Source: three-view drawing plus pictorial views. Frame: mm from the lowest corner of the part. Give positions to 0.01 mm unless a question says otherwise; leave off trailing zeros. Write each loop counter-clockwise with the first axis right and the second up, starting at its lowest first coordinate (ties: lowest second). Pieces come first, ordered by that corner, then holes. Notation, with made-up numbers: (77, -11) -> (81, -11) arc R18 cw to (81, 0) -> close; hole circle Ø2 at (50, 70). An arc over 180 degrees is marked (long way). Answer in a Markdown table with one row per item. Add a question column.
Item 1: Section query A-A on z = 100. Output: boundary loops of the cut face in (x, y), plus the area to 3 significant figures.
Item 2: Section query B-B on x = 114. Output: boundary loops of the cut face in (y, z).
Item 3: Section query C-C on y = 3.5. State how many separate pieces and enclosed holes the cut face has, plus the area to 3 significant figures.
Item 4: First-contact query: P1, Ø1.9, axis at y = 9.5, z = 195.5, coming from the -X side; P2, Ø1.5, axis at y = 6, z = 163, coming from the +X side; P3, Ø2, axis at y = 3.5, z = 147, coming from the +X side; P4, Ø6, axis at x = 37.27, z = 12.5, coming from the -Y side. Flat tips, straight axial feed; report the tip coordinate or a pass-through.
Item 5: Section query D-D on x = 76.5. Output: boundary loops of the cut face in (y, z).
Item 6: Material intervals for probe 1 along Z at (x, y) = (28, 5.5); probe 2 along Z at (x, y) = (114, 3.75); probe 3 along X at (y, z) = (9, 100), sorted ascending. Write a range as from..to.
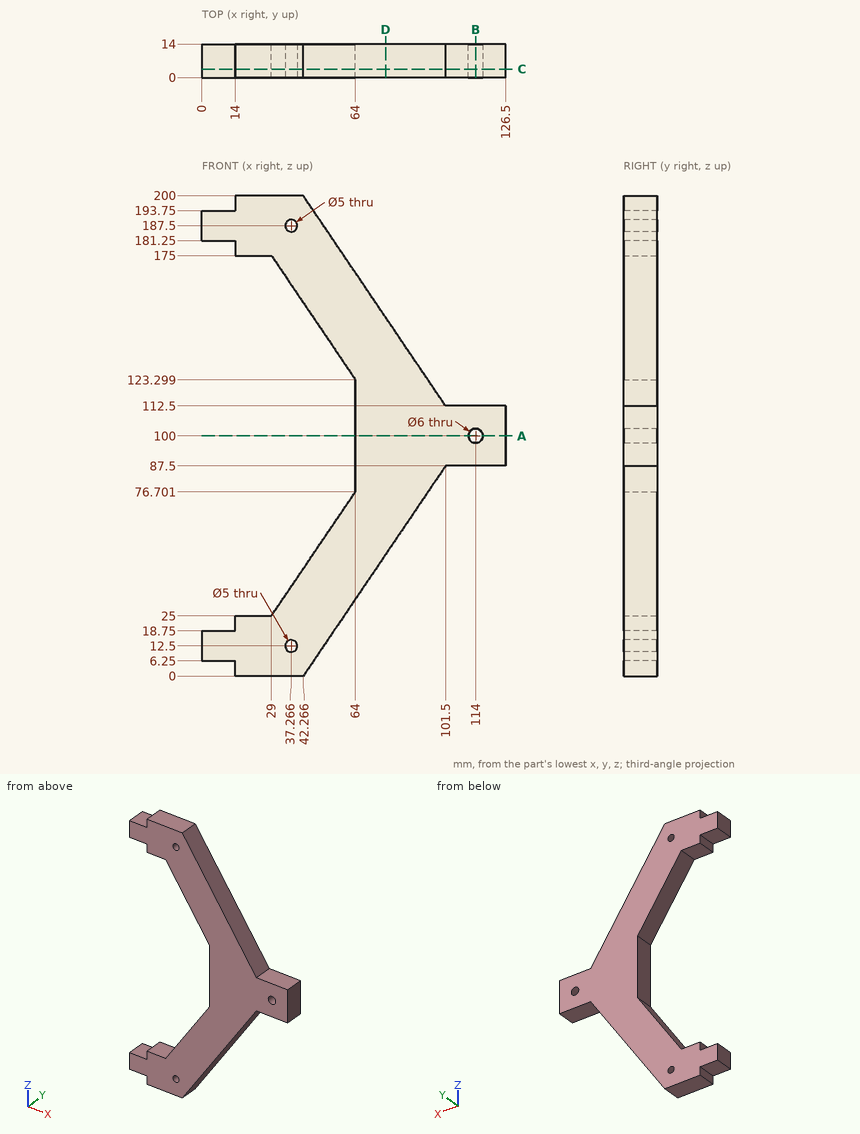
Findings below:
| question | item | result |
|---|---|---|
| 1 | outline | (64, 0) -> (111, 0) -> (111, 14) -> (64, 14) -> close; (117, 0) -> (126.5, 0) -> (126.5, 14) -> (117, 14) -> close |
| 1 | area | 791 mm^2 |
| 2 | outline | (0, 87.5) -> (14, 87.5) -> (14, 97) -> (0, 97) -> close; (0, 103) -> (14, 103) -> (14, 112.5) -> (0, 112.5) -> close |
| 3 | separate pieces | 1 |
| 3 | enclosed holes | 3 |
| 3 | area | 7,530 mm^2 |
| 4 | P1 | stops at x = 14 |
| 4 | P2 | stops at x = 67.82 |
| 4 | P3 | stops at x = 78.82 |
| 4 | P4 | stops at y = 0 |
| 5 | outline | (0, 50.57) -> (14, 50.57) -> (14, 149.43) -> (0, 149.43) -> close |
| 6 | probe 1 | z = 0..25, 175..200 |
| 6 | probe 2 | z = 87.5..97, 103..112.5 |
| 6 | probe 3 | x = 64..111, 117..126.5 |
